Work out the finished part from the listing and answer in its coordinate system (mm). A direction names the side the tool comes from. Round coordinates to 2 decimals unless told otherwise and drop trailing zeros. Write each loop counter-clockwise with the first axis right and the second up, starting at its lowest first coordinate (ties: lowest second). Pieces come first, ordered by that corner, then holes. Notation, with made-up numbers: (60.5, -15.75) - (87.5, -15.75) arc R23 ccw to (87.5, -6.75) - close; hole circle Ø1 at (21, -26). An arc over 180 degrees is marked (long way). Answer as a JSON object with one key per item and string values.
```python
from build123d import *

# Parameters (mm, degrees)
MAIN_DEPTH              = 55
FIXING_DEPTH            = 52.577177515
ESQUISSE4_R             = 1.6
ENL_V_MAT_EXTRU_6_DEPTH = 14
CENTRAL_HOLE_DEPTH      = 22


with BuildPart() as part:
    # Esquisse1 → Main (new body, symmetric)
    with BuildSketch(Plane.XY):
        Polygon((0, 0), (13, 0), (13, 13), (90, 26.577177515), (90, 51.577177515), (0, 35.707749251), align=None)
    extrude(amount=MAIN_DEPTH, both=True)

    # Esquisse3 → Fixing (cut, through all)
    with BuildSketch(Plane(origin=(-3.294458096, 0, 0), x_dir=(1, 0, 0), z_dir=(0, 1, 0))):
        Polygon((3.294458096, 45), (6.844458096, 45), (6.844458096, 46), (9.744458096, 46), (9.744458096, 45), (13.294458096, 45), (13.294458096, 48.55), (12.294458096, 48.55), (12.294458096, 51.45), (13.294458096, 51.45), (13.294458096, 55), (3.294458096, 55), align=None)
    fixing = extrude(amount=FIXING_DEPTH, mode=Mode.SUBTRACT)

    # Esquisse4 → Enlèv. mat.-Extru.6 (cut, through all)
    with BuildSketch(Plane(origin=(13, 0, 0), x_dir=(0, 0, -1), z_dir=(1, 0, 0))):
        with Locations((-50, 5)):
            Circle(ESQUISSE4_R)
    enl_v_mat_extru_6 = extrude(amount=-ENL_V_MAT_EXTRU_6_DEPTH, mode=Mode.SUBTRACT)

    # Symétrie1: Fixing, Enlèv. mat.-Extru.6 across plane
    add(fixing.mirror(Plane.XY), mode=Mode.SUBTRACT)
    add(enl_v_mat_extru_6.mirror(Plane.XY), mode=Mode.SUBTRACT)

    # Esquisse2 → Central Hole (cut)
    with BuildSketch(Plane(origin=(-6.106384758, 34.631028863, 0), x_dir=(0.984807753, 0.173648178, 0), z_dir=(-0.173648178, 0.984807753, 0))):
        Polygon((97.588980656, 52.5), (97.588980656, -52.5), (19.354851705, -42.5), (-3.799414414, -42.5), (-3.799414414, 42.5), (19.354851705, 42.5), align=None)
    extrude(amount=-CENTRAL_HOLE_DEPTH, mode=Mode.SUBTRACT)


solid = part.part
```
Item 1: Determine the mould class of faces 1 (the cylindrical face through (11.03, 5.07, -51.6)), 2 (the flat face through (9, 21, 50)), 3 (the flat face through (8, 18, 45)) for opening direction X: pulls with the +X half, pulls with the -X half, needs draft (parallel to the pull), parting line crosses it, or undercut.
Results found:
{"face 1": "needs draft", "face 2": "pulls with the -X half", "face 3": "undercut"}
Item 2: For faces 4 (the flat face through (5, 18, 46)), 5 (the flat face through (7, 26, 42.5)), 6 (the flat face through (10, 18, -53)), 7 (the flat face through (13, 6, 1)), 8 (the flat face through (10, 18, 47)), determine the directions among +Z, -Z, +X, -X, +Y, -Y from which every point of the face is accessible in a straight line to the end or side of a thin tool.
Results found:
{"face 4": "+Z, -X, +Y, -Y", "face 5": "-X, +Y", "face 6": "-Z, -X, +Y, -Y", "face 7": "+Z, -Z, +X, -Y", "face 8": "+Y, -Y"}
Item 3: Consider line 1 along Y through (x, z) = (11, 50); line 2 along Z through (x, y) = (20, 39); line 3 along Z through (x, y) = (60.5, 38.5). Determine where each line is inside the solid, lowest interval first.
Results found:
{"line 1": "0 to 3.4, 6.6 to 37.65", "line 2": "-55 to -43.41, 43.41 to 55", "line 3": "-55 to -48.5, 48.5 to 55"}
Item 4: Each of these flat-tipped pins is pushed along its axis until it touches: P1, Ø4, axis at y = 7.5, z = 13, coming from the +X side; P2, Ø4, axis at x = 7.5, y = 23.5, coming from the -Z side; P3, Ø1, axis at x = 63.5, z = -39.5, coming from the -Y side; P4, Ø3, axis at y = 5, z = 50, coming from the -X side. Where does it stop, or does it pass through?
Results found:
{"P1": "x = 13", "P2": "z = -51.45", "P3": "y = 21.82", "P4": "through"}
Item 5: A cutting plane is placed at D-D (z = 50). Write down the section's boundary in (x, y).
Results found:
{"outline": "(9, 0) - (13, 0) - (13, 3.4) - (9, 3.4) - close; (9, 6.6) - (13, 6.6) - (13, 13) - (90, 26.58) - (90, 29.24) - (74.56, 26.52) - (70.74, 48.18) - (9, 37.29) - close"}
Item 6: A cutting plane is placed at B-B (z = 17.5). Write down the section's boundary in (x, y), and give its area (3 significant figures).
Results found:
{"outline": "(0, 0) - (13, 0) - (13, 13) - (90, 26.58) - (90, 29.24) - (0, 13.37) - close", "area": "394 mm²"}
Item 7: A cutting plane is placed at A-A (x = 51). Write down the section's boundary in (y, z), and give its area (3 significant figures).
Results found:
{"outline": "(19.7, -55) - (44.7, -55) - (44.7, -47.44) - (22.36, -46.94) - (22.36, 46.94) - (44.7, 47.44) - (44.7, 55) - (19.7, 55) - close", "area": "642 mm²"}
